Geometry: final body of the model. Coordinates: model frame, mm. Round coordinates to 2 decimals unless told otherwise and drop trailing zeros. Loops run counter-clockwise (first coordinate to the right, second up) from the corner with the lowest first, then second, coordinate; pieces in that order, holes last. Notation, with made-up numbers: M 4,32 L 17,32 A20 ccw 17,66 Z; hole C -2,88 d5. An arc over 180 degrees is marked long. Return JSON: item names as keys, results as strings.
from build123d import *

# Parameters (mm, degrees)
SALIENTE_EXTRUIR1_DEPTH                        = 100
CSK_FOR_M3_FLAT_HEAD_MACHINE_SCREW1_AT_2_COUNT = 2
CSK_FOR_M3_FLAT_HEAD_MACHINE_SCREW1_AT_2_PITCH = 90
CSK_FOR_M3_FLAT_HEAD_MACHINE_SCREW1_AT_3_COUNT = 2
CSK_FOR_M3_FLAT_HEAD_MACHINE_SCREW1_AT_3_PITCH = 95.51963149
CSK_FOR_M3_FLAT_HEAD_MACHINE_SCREW1_AT_4_COUNT = 2
CSK_FOR_M3_FLAT_HEAD_MACHINE_SCREW1_AT_4_PITCH = 32
CROQUIS4_W                                     = 6.5
CROQUIS4_H                                     = 3.5
CORTAR_EXTRUIR3_DEPTH                          = 121.957265181
CROQUIS8_W                                     = 13.5
CROQUIS8_H                                     = 7.5
CORTAR_EXTRUIR4_DEPTH                          = 2.5
CORTAR_EXTRUIR5_DEPTH                          = 1
CROQUIS12_W                                    = 67.9
CROQUIS12_H                                    = 8.529184672
CORTAR_EXTRUIR6_DEPTH                          = 1


with BuildPart() as part:
    # Croquis1 → Saliente-Extruir1 (new body)
    with BuildSketch(Plane(origin=(0, 0, 0), x_dir=(0, 0, -1), z_dir=(1, 0, 0))):
        Polygon((0, 0), (67.9, 0), (67.9, 4.5), (16.794228634, 4.5), align=None)
    extrude(amount=SALIENTE_EXTRUIR1_DEPTH)

    # Croquis3 → CSK for M3 Flat Head Machine Screw1 (revolve, cut)
    with BuildSketch(Plane(origin=(95, 0, -59.42), x_dir=(0, 0, -1), z_dir=(1, 0, 0))):
        Polygon((0, 0), (0, 4.5), (1.7, 4.5), (1.7, 2.741033263), (4, 0), align=None)
    csk_for_m3_flat_head_machine_screw1 = revolve(axis=Axis((95, -6.35, -59.42), (0, 1, 0)), mode=Mode.SUBTRACT)

    # CSK for M3 Flat Head Machine Screw1 at 2: CSK for M3 Flat Head Machine Screw1 ×2
    with Locations(*[(-i * CSK_FOR_M3_FLAT_HEAD_MACHINE_SCREW1_AT_2_PITCH, 0, 0) for i in range(1, CSK_FOR_M3_FLAT_HEAD_MACHINE_SCREW1_AT_2_COUNT)]):
        add(csk_for_m3_flat_head_machine_screw1, mode=Mode.SUBTRACT)

    # CSK for M3 Flat Head Machine Screw1 at 3: CSK for M3 Flat Head Machine Screw1 ×2
    with Locations(*[Vector(-0.9422146902791427, 0, 0.33500966765479934) * (i * CSK_FOR_M3_FLAT_HEAD_MACHINE_SCREW1_AT_3_PITCH) for i in range(1, CSK_FOR_M3_FLAT_HEAD_MACHINE_SCREW1_AT_3_COUNT)]):
        add(csk_for_m3_flat_head_machine_screw1, mode=Mode.SUBTRACT)

    # CSK for M3 Flat Head Machine Screw1 at 4: CSK for M3 Flat Head Machine Screw1 ×2
    with Locations(*[(0, 0, i * CSK_FOR_M3_FLAT_HEAD_MACHINE_SCREW1_AT_4_PITCH) for i in range(1, CSK_FOR_M3_FLAT_HEAD_MACHINE_SCREW1_AT_4_COUNT)]):
        add(csk_for_m3_flat_head_machine_screw1, mode=Mode.SUBTRACT)

    # Croquis4 → Cortar-Extruir3 (cut, through all)
    with BuildSketch(Plane(origin=(0, 4.5, 0), x_dir=(1, 0, 0), z_dir=(0, 1, 0))):
        with Locations((15, 17.19)):
            Rectangle(CROQUIS4_W, CROQUIS4_H)
        with Locations((85, 17.19)):
            Rectangle(CROQUIS4_W, CROQUIS4_H)
    extrude(amount=-CORTAR_EXTRUIR3_DEPTH, mode=Mode.SUBTRACT)

    # Croquis8 → Cortar-Extruir4 (cut)
    with BuildSketch(Plane(origin=(0, 4.5, 0), x_dir=(1, 0, 0), z_dir=(0, 1, 0))):
        with Locations((15, 17.19)):
            Rectangle(CROQUIS8_W, CROQUIS8_H)
        with Locations((85, 17.19)):
            Rectangle(CROQUIS8_W, CROQUIS8_H)
    extrude(amount=-CORTAR_EXTRUIR4_DEPTH, mode=Mode.SUBTRACT)

    # Croquis11 → Cortar-Extruir5 (cut)
    with BuildSketch(Plane(origin=(100, 0, 0), x_dir=(0, 0, -1), z_dir=(1, 0, 0))):
        Polygon((0, 0), (67.9, 0), (67.9, 7.340226628), (-0.455473411, 7.340226628), align=None)
    extrude(amount=-CORTAR_EXTRUIR5_DEPTH, mode=Mode.SUBTRACT)

    # Croquis12 → Cortar-Extruir6 (cut)
    with BuildSketch(Plane.ZY):
        with Locations((-33.95, 4.264592336)):
            Rectangle(CROQUIS12_W, CROQUIS12_H)
    extrude(amount=-CORTAR_EXTRUIR6_DEPTH, mode=Mode.SUBTRACT)


solid = part.part
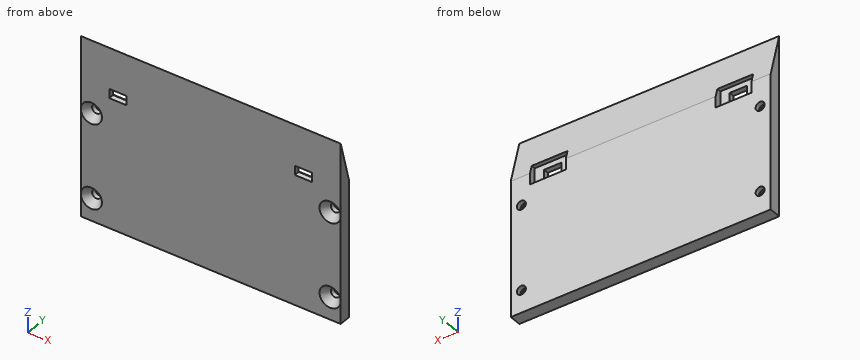
Q1. Pin query (flat end, axial travel): pin 1 (6 mm diameter, centred on x = 84, z = -17, fed in from +Y); pin 2 (2 mm diameter, centred on x = 95, z = -59.42, fed in from -Y). Return the tip coordinate at first contact, or that it passes through.
Determined:
{"pin 1": "stops at y = 2", "pin 2": "passes through"}
Q2. Section query A-A (x = 95). Output: boundary loops of the cut face in (y, z), plus the area to 3 significant figures.
Determined:
{"outline": "M 0,-67.9 L 4.5,-67.9 L 4.5,-61.12 L 2.74,-61.12 L 0,-63.42 Z; M 0,-55.42 L 2.74,-57.72 L 4.5,-57.72 L 4.5,-29.12 L 2.74,-29.12 L 0,-31.42 Z; M 0,-23.42 L 2.74,-25.72 L 4.5,-25.72 L 4.5,-16.79 L 0,0 Z", "area": "225 mm^2"}
Q3. Section query B-B (z = -12). Output: boundary loops of the cut face in (x, y).
Determined:
{"outline": "M 1,0 L 99,0 L 99,3.22 L 1,3.22 Z"}
Q4. Section query C-C (x = 61.5). Output: boundary loops of the cut face in (y, z), plus the area to 3 significant figures.
Determined:
{"outline": "M 0,-67.9 L 4.5,-67.9 L 4.5,-16.79 L 0,0 Z", "area": "268 mm^2"}
Q5. Material intervals for L1, parallel to X at y = 3.85, z = -27.42; L2, parallel to Y at x = 74, z = -15.5; L3, parallel to Y at x = 92.5, z = -16.5, sorted ascending.
Determined:
{"L1": "x = 1 to 3.3, 6.7 to 93.3, 96.7 to 99", "L2": "y = 0 to 4.15", "L3": "y = 0 to 4.42"}
